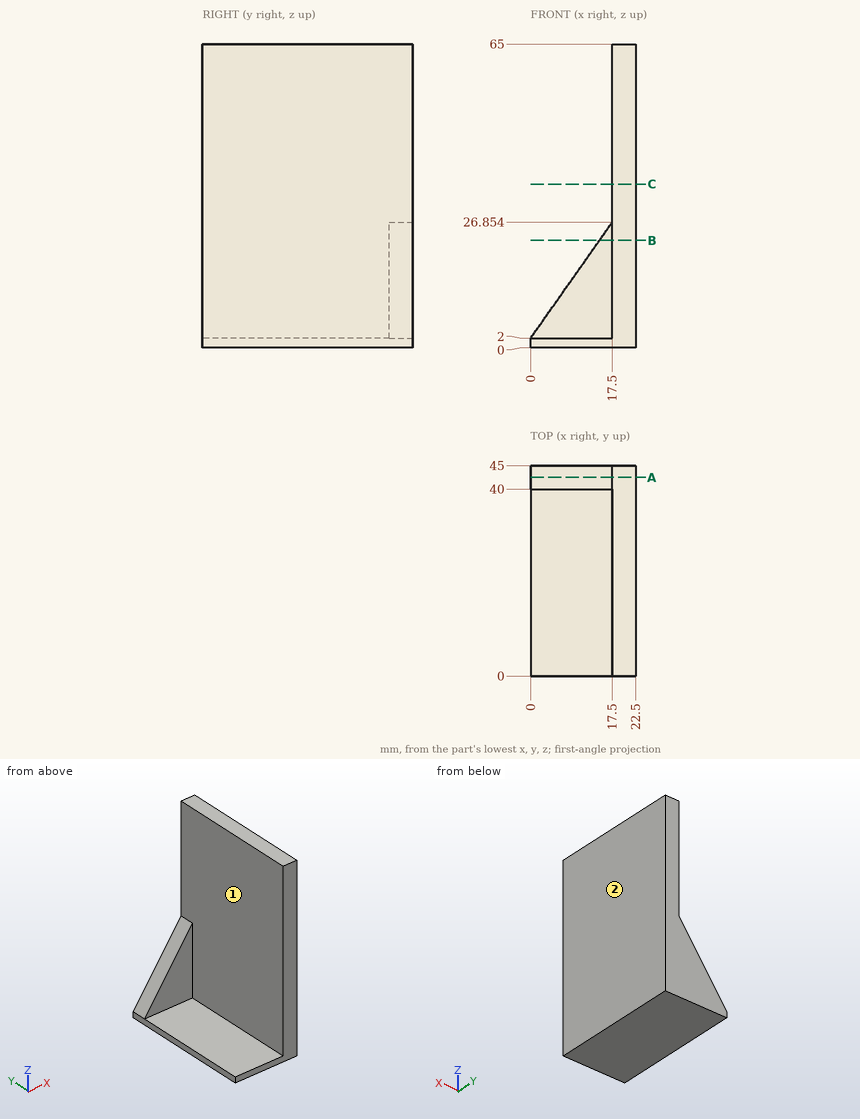
Verification items for this drawing (mm, ordinates from the low corner). A direction names the side the tool comes from. Coordinates: 2 decimals unless noted, no trailing zeros. Order: outer loops, then holes, each group sorted by start corner. A loop starts at its lowest first (then second) coordinate and runs counter-clockwise, first axis right, second up. Notation, with made-up numbers: (-13.75, 5) - (30.25, 5) arc R6 ccw to (30.25, 10) - close; hole circle Ø1 at (10, 81.5). An arc over 180 degrees is marked (long way). Answer as a JSON object with one key per item and string values. Group by question number.
Item 1: Sectioned sample at A-A, the plane y = 42.5. Record the cut outline in (x, z).
Item 2: Scan lines: probe 1 along X at (y, z) = (2.5, 28); probe 2 along Y at (x, z) = (9.5, 11.5); probe 3 along Z at (x, y) = (8.5, 16.5). Record each from-to range of solid material in increasing order.
Item 3: Sectioned sample at B-B, the plane z = 23. Record the cut outline in (x, y), and give its area (3 significant figures).
Item 4: Depth check by flat-ended pin: pin 1 Ø5 at (x, z) = (20, 51.5) entering from -Y; pin 2 Ø9 at (x, z) = (12.5, 16.5) entering from -Y; pin 3 Ø5 at (y, z) = (22, 38) entering from -X; pin 4 Ø12 at (x, z) = (5, 28.5) entering from -Y. Enter the tip coordinate at first touch or a pass-through.
Item 5: Tool access check on the marked faces 1 and 2. Record the directions out of +Z, -Z, +X, -X, +Y, -Y that give a thin tool (end or side, any length) a straight path to the whole face; none if there is none.
Item 6: Sectioned sample at C-C, the plane z = 35. Record the cut outline in (x, y).
Resolved:
{
 "1": {"outline": "(0, 0) - (22.5, 0) - (22.5, 65) - (17.5, 65) - (17.5, 26.85) - (0, 2) - close"},
 "2": {"probe 1": "17.5 to 22.5", "probe 2": "40 to 45", "probe 3": "0 to 2"},
 "3": {"outline": "(14.79, 40) - (17.5, 40) - (17.5, 0) - (22.5, 0) - (22.5, 45) - (14.79, 45) - close", "area": "239 mm^2"},
 "4": {"pin 1": "y = 0", "pin 2": "y = 40", "pin 3": "x = 17.5", "pin 4": "through"},
 "5": {"face 1": "+Z, -X, -Y", "face 2": "+Z, -Z, +X, +Y, -Y"},
 "6": {"outline": "(17.5, 0) - (22.5, 0) - (22.5, 45) - (17.5, 45) - close"}
}
